For this review, use the dimensioned drawing (mm, ordinates from the lowest corner) and the shaded views. A direction names the side the tool comes from. Round coordinates to 2 decimals unless told otherwise and drop trailing zeros. Write each loop counter-clockwise with the first axis right and the second up, starting at its lowest first coordinate (ties: lowest second). Pieces come first, ordered by that corner, then holes. Notation, with made-up numbers: (26.5, -33.75) - (37.5, -33.75) arc R8 ccw to (37.5, -21.75) - close; hole circle Ø1 at (78.25, -17.75). An arc over 180 degrees is marked (long way). Return JSON: item names as keys, results as strings.
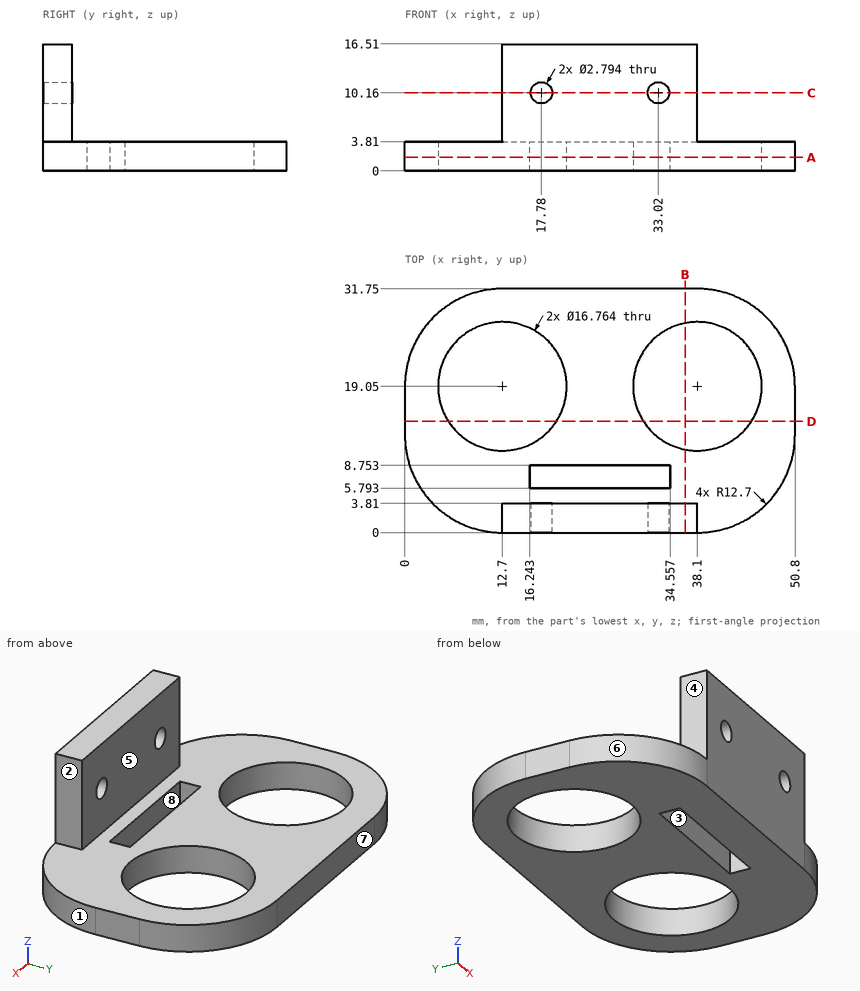
(1) Mouldability with a two-part tool opening along Y and no side actions: class the marked faces 6, 7 and 8 as released by +Y, released by -Y, zero draft, split by the parting line, or undercut.
Filled in:
{"face 6": "released by -Y", "face 7": "released by +Y", "face 8": "undercut"}
(2) Add section A-A (z = 1.75). Write out the cut boundary in (x, y), plus the area to 3 significant figures.
Filled in:
{"outline": "(0, 12.7) arc R12.7 ccw to (12.7, 0) - (38.1, 0) arc R12.7 ccw to (50.8, 12.7) - (50.8, 19.05) arc R12.7 ccw to (38.1, 31.75) - (12.7, 31.75) arc R12.7 ccw to (0, 19.05) - close; hole circle Ø16.76 at (12.7, 19.05); hole (16.24, 5.79) - (34.56, 5.79) - (34.56, 8.75) - (16.24, 8.75) - close; hole circle Ø16.76 at (38.1, 19.05)", "area": "979 mm2"}
(3) Clearance check with flat-ended pins moving along their axes: pin 1 Ø1.9 at (x, z) = (24, 2) entering from -Y; pin 2 Ø1.9 at (y, z) = (1, 13) entering from +X; pin 3 Ø3.5 at (x, z) = (17.78, 10.16) entering from +Y; pin 4 Ø1.5 at (y, z) = (8, 2.5) entering from -X. State where each tip first meets the part, or that it passes through.
Filled in:
{"pin 1": "stops at y = 0", "pin 2": "stops at x = 38.1", "pin 3": "stops at y = 3.81", "pin 4": "stops at x = 0.63"}
(4) Add section D-D (y = 14.5). Write out the cut boundary in (x, z).
Filled in:
{"outline": "(0, 0) - (5.66, 0) - (5.66, 3.81) - (0, 3.81) - close; (19.74, 0) - (31.06, 0) - (31.06, 3.81) - (19.74, 3.81) - close; (45.14, 0) - (50.8, 0) - (50.8, 3.81) - (45.14, 3.81) - close"}
(5) Add section C-C (z = 10.16). Write out the cut boundary in (x, y).
Filled in:
{"outline": "(12.7, 0) - (16.38, 0) - (16.38, 3.81) - (12.7, 3.81) - close; (19.18, 0) - (31.62, 0) - (31.62, 3.81) - (19.18, 3.81) - close; (34.42, 0) - (38.1, 0) - (38.1, 3.81) - (34.42, 3.81) - close"}
(6) For the marked faces 1, 2, 3, 4 and 5, list the 3-axis set-ups (+Z, -Z, +X, -X, +Y, -Y) from which the entire face can be reached by the end or side of a thin tool; tool diameter is ignored.
Filled in:
{"face 1": "+Z, -Z, +X, -Y", "face 2": "+Z, +X, +Y, -Y", "face 3": "+Z, -Z", "face 4": "+Z, -X, +Y, -Y", "face 5": "+Z, +X, -X, +Y"}
(7) Wall thickness on line 1 (Y direction, x = 38.1, z = 1.3); line 2 (Z direction, x = 33.02, y = 2.65); line 3 (Z direction, x = 31.5, y = 27.5): over which ranges is each line inside the solid? List them lowest first.
Filled in:
{"line 1": "y = 0 to 10.67, 27.43 to 31.75", "line 2": "z = 0 to 8.76, 11.56 to 16.51", "line 3": "z = 0 to 3.81"}
(8) Add section B-B (x = 36.5). Write out the cut boundary in (y, z).
Filled in:
{"outline": "(0, 0) - (10.82, 0) - (10.82, 3.81) - (3.81, 3.81) - (3.81, 16.51) - (0, 16.51) - close; (27.28, 0) - (31.75, 0) - (31.75, 3.81) - (27.28, 3.81) - close"}
